Source: CAD feature listing. Evaluate the final solid. Frame: model axes, mm. A direction names the side the tool comes from. Round coordinates to 2 decimals unless told otherwise and drop trailing zeros. Order: outer loops, then holes, each group sorted by start corner. A loop starts at its lowest first (then second) coordinate and runs counter-clockwise, first axis right, second up. Notation, with made-up numbers: M 83.25,-22 L 128.25,-22 A30 ccw 128.25,10 Z; hole C 44.25,44 d1. An arc over 180 degrees is marked long. Answer as CSV lines item,"result". Start each with the question number.
Item 1: First-contact query: P1, Ø3, axis at x = 21.5, y = 12.5, coming from the +Z side; P2, Ø23, axis at x = 1, z = 1, coming from the +Y side; P3, Ø10, axis at y = 33, z = 22.5, coming from the -X side. Flat tips, straight axial feed; report the tip coordinate or a pass-through.
Item 2: Section query D-D on y = 35. Return the cut outline in (x, z).
Item 3: Section query B-B on y = 13.5. Return the cut outline in (x, z), plus the area to 3 significant figures.
Item 4: Section query A-A on x = 0. Return the cut outline in (y, z), plus the area to 3 significant figures.
Item 5: Line query: line 1 (X direction, y = 6.1, z = 0); line 2 (X direction, y = 27.5, z = 0). Output: solid intervals per line, ascending. Write a range as [from, to].
Item 6: Section query C-C on z = 12.5. Return the cut outline in (x, y).
Item 7: Pull-direction query (X, two-part tool) for faces 4 (the face through (-16.84, 7.46, -15.44)), 5 (the face through (-29.97, 27.88, -1.32)), 6 (the face through (-7, 55, 22)); classes: +X half, -X half, draft (parallel to the pull), parting line (faces both ways), or undercut.
Item 8: Set-up query: faces 1 (the face through (0, 0, 0)), 2 (the face through (-22.826, 34.72, -0.991)), 3 (the face through (-23, 15, 0)). Return all of +Z, -Z, +X, -X, +Y, -Y with unobstructed straight access to the full face (end or side cutting, diameter ignored); none if empty.
from build123d import *

# Parameters (mm, degrees)
SKETCH6_R          = 1
CUT_EXTRUDE4_DEPTH = 40


with BuildPart() as part:
    # Sketch4 → Revolve2 (revolve)
    with BuildSketch(Plane.XY):
        Polygon((0, 0), (30, 0), (30, 55), (22.847682119, 55), (22.847682119, 15), (23.847682119, 15), (23.847682119, 10), (22.847682119, 10), (22.847682119, 5), (0, 5), align=None)
    revolve(axis=Axis((0, -1100.033698247, 0), (0, 1, 0)))

    # Sketch6 → Cut-Extrude4 (cut)
    with BuildSketch(Plane(origin=(0, 55, 0), x_dir=(1, 0, 0), z_dir=(0, 1, 0))):
        with Locations((22.847682119, 0)):
            Circle(SKETCH6_R)
    extrude(amount=-CUT_EXTRUDE4_DEPTH, mode=Mode.SUBTRACT)


solid = part.part
Results:
1,P1,"z = 22.36"
1,P2,"y = 5"
1,P3,"x = -24.37"
2,outline,"C 0,0 d60; hole M 22.83,-1 A1 ccw long 22.83,1 A22.85 ccw long Z"
3,outline,"C 0,0 d60; hole C 0,0 d47.7"
3,area,"1,040 mm^2"
4,outline,"M 0,-30 L 55,-30 L 55,-22.85 L 15,-22.85 L 15,-23.85 L 10,-23.85 L 10,-22.85 L 5,-22.85 L 5,22.85 L 10,22.85 L 10,23.85 L 15,23.85 L 15,22.85 L 55,22.85 L 55,30 L 0,30 Z"
4,area,"1,010 mm^2"
5,line 1,"[-30, -22.85], [22.85, 30]"
5,line 2,"[-30, -22.85], [23.85, 30]"
6,outline,"M -27.27,0 L 27.27,0 L 27.27,55 L 19.13,55 L 19.13,15 L 20.31,15 L 20.31,10 L 19.13,10 L 19.13,5 L -19.13,5 L -19.13,10 L -20.31,10 L -20.31,15 L -19.13,15 L -19.13,55 L -27.27,55 Z"
7,face 4,"undercut"
7,face 5,"parting line"
7,face 6,"draft"
8,face 1,"+Z, -Z, +X, -X, -Y"
8,face 2,"+Y"
8,face 3,"none"
